Geometry: final body of the model. Coordinates: model frame, mm. Face numbers are marked on the shaded views. A direction names the side the tool comes from. Give positions to 0.01 mm unless a question says otherwise; leave off trailing zeros. Write each loop counter-clockwise with the first axis right and the second up, starting at its lowest first coordinate (ties: lowest second). Pieces come first, ordered by that corner, then holes. Notation, with made-up numbers: M 62,-11 L 108,-11 A22 ccw 108,21 Z; hole C 9.5,31.25 d3. An arc over 180 degrees is marked long. Answer as a JSON object with one key per item and string values.
from build123d import *

# Parameters (mm, degrees)
SKETCH1_W           = 175
SKETCH1_H           = 6.75
BOSS_EXTRUDE1_DEPTH = 6.5
SKETCH2_W           = 10
SKETCH2_H           = 6.75
BOSS_EXTRUDE2_DEPTH = 7.5
SKETCH5_R           = 3.175
CUT_EXTRUDE2_DEPTH  = 10
LPATTERN1_COUNT     = 6
LPATTERN1_PITCH     = 25
SKETCH6_R           = 3.175
BOSS_EXTRUDE4_DEPTH = 6.75
LPATTERN2_COUNT     = 6
LPATTERN2_PITCH     = 25
BOSS_EXTRUDE5_DEPTH = 6.5
BOSS_EXTRUDE6_DEPTH = 3
SKETCH10_R          = 2.575
CUT_EXTRUDE4_DEPTH  = 2
CUT_EXTRUDE5_DEPTH  = 18
SKETCH12_R          = 1
CUT_EXTRUDE6_DEPTH  = 10


with BuildPart() as part:
    # Sketch1 → Boss-Extrude1 (new body)
    with BuildSketch(Plane(origin=(0, 0, 0), x_dir=(1, 0, 0), z_dir=(0, 1, 0))):
        with Locations((87.5, -3.375)):
            Rectangle(SKETCH1_W, SKETCH1_H)
    extrude(amount=BOSS_EXTRUDE1_DEPTH)

    # Sketch2 → Boss-Extrude2 (add)
    with BuildSketch(Plane(origin=(0, 6.5, 0), x_dir=(1, 0, 0), z_dir=(0, 1, 0))):
        with Locations((5, -3.375)):
            Rectangle(SKETCH2_W, SKETCH2_H)
    boss_extrude2 = extrude(amount=BOSS_EXTRUDE2_DEPTH)

    # Sketch5 → Cut-Extrude2 (cut)
    with BuildSketch(Plane.XY.offset(6.75)):
        with Locations((5, 8.75)):
            Circle(SKETCH5_R)
    cut_extrude2 = extrude(amount=-CUT_EXTRUDE2_DEPTH, mode=Mode.SUBTRACT)

    # LPattern1: Boss-Extrude2, Cut-Extrude2 ×6
    with Locations(*[(i * LPATTERN1_PITCH, 0, 0) for i in range(1, LPATTERN1_COUNT)]):
        add(boss_extrude2)
        add(cut_extrude2, mode=Mode.SUBTRACT)

    # Sketch6 → Boss-Extrude4 (add)
    with BuildSketch(Plane.XY.offset(6.75)):
        Polygon((138.660254038, 8.75), (138.660254038, 0), (121.339745962, 0), (121.339745962, 8.75), (125.669872981, 16.25), (134.330127019, 16.25), align=None)
        with Locations((130, 8.75)):
            Circle(SKETCH6_R, mode=Mode.SUBTRACT)
    boss_extrude4 = extrude(amount=-BOSS_EXTRUDE4_DEPTH)

    # LPattern2: Boss-Extrude4 ×6
    with Locations(*[(-i * LPATTERN2_PITCH, 0, 0) for i in range(1, LPATTERN2_COUNT)]):
        add(boss_extrude4)

    # Sketch7 → Boss-Extrude5 (add)
    with BuildSketch(Plane(origin=(0, 6.5, 0), x_dir=(1, 0, 0), z_dir=(0, 1, 0))):
        Polygon((172.113248654, -8.375), (177.886751346, -8.375), (178.824945533, -6.75), (182.289047149, -6.75), (179.618802154, -11.375), (170.381197846, -11.375), (165.762395693, -3.375), (170.381197846, 4.625), (179.618802154, 4.625), (181.350852961, 1.625), (177.886751346, 1.625), (172.113248654, 1.625), (169.226497308, -3.375), align=None)
    extrude(amount=-BOSS_EXTRUDE5_DEPTH)

    # Sketch9 → Boss-Extrude6 (add)
    with BuildSketch(Plane(origin=(0, 0, 0), x_dir=(-1, 0, 0), z_dir=(0, -1, 0))):
        Polygon((-169.226497308, -3.375), (-172.113248654, 1.625), (-177.886751346, 1.625), (-181.350852961, 1.625), (-184.237604307, -3.375), (-182.289047149, -6.75), (-178.824945533, -6.75), (-177.886751346, -8.375), (-172.113248654, -8.375), align=None)
    extrude(amount=-BOSS_EXTRUDE6_DEPTH)

    # Sketch10 → Cut-Extrude4 (cut)
    with BuildSketch(Plane(origin=(0, 0, 0), x_dir=(-1, 0, 0), z_dir=(0, -1, 0))):
        with Locations((-175, -3.375)):
            Circle(SKETCH10_R)
    extrude(amount=-CUT_EXTRUDE4_DEPTH, mode=Mode.SUBTRACT)

    # Sketch11 → Cut-Extrude5 (cut)
    with BuildSketch(Plane(origin=(0, 3, 0), x_dir=(1, 0, 0), z_dir=(0, 1, 0))):
        Polygon((180.773502692, -3.375), (177.886751346, 1.625), (172.113248654, 1.625), (169.226497308, -3.375), (172.113248654, -8.375), (177.886751346, -8.375), align=None)
    extrude(amount=CUT_EXTRUDE5_DEPTH, mode=Mode.SUBTRACT)

    # Sketch12 → Cut-Extrude6 (cut)
    with BuildSketch(Plane(origin=(0, 3, 0), x_dir=(1, 0, 0), z_dir=(0, 1, 0))):
        with Locations((175, -3.375)):
            Circle(SKETCH12_R)
    extrude(amount=-CUT_EXTRUDE6_DEPTH, mode=Mode.SUBTRACT)


solid = part.part
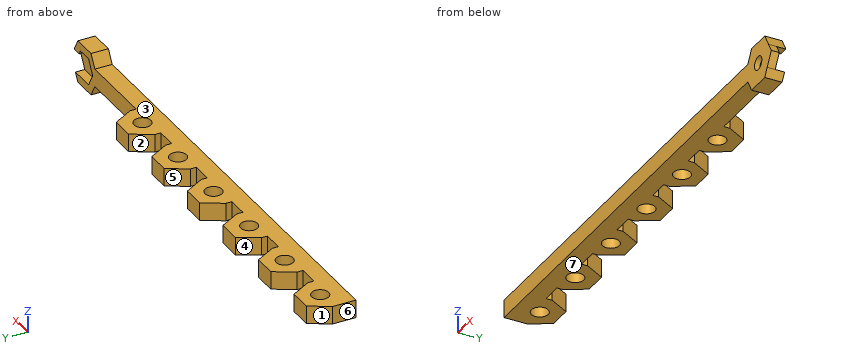
1) Set-up query: the marked faces 1, 2 and 3. Return all of +Z, -Z, +X, -X, +Y, -Y with unobstructed straight access to the full face (end or side cutting, diameter ignored); none if empty.
Geometry check:
{"face 1": "+Z, -Z, -X, +Y", "face 2": "+Z, -Z, +Y", "face 3": "+Z, -X, +Y, -Y"}
2) Cut plane B-B on x = 103.5. Return loops of the section in (y, z).
Geometry check:
{"outline": "M 0,0 L 5.95,0 L 5.95,6.75 L 0,6.75 Z; M 11.55,0 L 16.25,0 L 16.25,6.75 L 11.55,6.75 Z"}
3) Pull-direction query (X, two-part tool) for the marked faces 4, 5, 6 and 7; classes: pulls with the +X half, pulls with the -X half, needs draft (parallel to the pull), parting line crosses it, or undercut.
Geometry check:
{"face 4": "undercut", "face 5": "undercut", "face 6": "pulls with the -X half", "face 7": "needs draft"}
4) Contact query for flat-ended pins moving along their axis: P1, Ø8, axis at y = 10, z = 9, coming from the +X side; P2, Ø5.5, axis at x = 69.5, z = 2, coming from the +Y side; P3, Ø5, axis at x = 109, z = 5.5, coming from the -Y side; P4, Ø4, axis at x = 130, y = 8.75, coming from the -Z side. Output: stop coordinate, or through.
Geometry check:
{"P1": "stops at x = 182.11", "P2": "stops at y = 10.33", "P3": "stops at y = 0", "P4": "passes through"}
5) Cut plane C-C on x = 66. Return loops of the section in (y, z), and give its area (3 significant figures).
Geometry check:
{"outline": "M 0,0 L 6.5,0 L 6.5,6.75 L 0,6.75 Z", "area": "43.9 mm2"}
6) Cut plane A-A on x = 30. Return loops of the section in (y, z) (3 decimals).
Geometry check:
{"outline": "M 0,0 L 5.575,0 L 5.575,6.75 L 0,6.75 Z; M 11.925,0 L 16.25,0 L 16.25,6.75 L 11.925,6.75 Z"}
7) Line query: line 1 (Y direction, x = 80, z = 4) (3 decimals); line 2 (Z direction, x = 175, y = 0.65) (3 decimals); line 3 (X direction, y = 15, z = 3.25). Output: solid intervals per line, ascending. Write a range as from..to.
Geometry check:
{"line 1": "y = 0..5.575, 11.925..16.25", "line 2": "z = -4.625..0.8, 5.95..11.375", "line 3": "x = -0.05..10.05, 24.95..35.05, 49.95..60.05, 74.95..85.05, 99.95..110.05, 124.95..135.05"}
